Build history of the part. All positions in model axes, mm. Face numbers are marked on the shaded views. A direction names the side the tool comes from. Give positions to 0.01 mm unless a question says otherwise; leave off trailing zeros. Loops run counter-clockwise (first coordinate to the right, second up) from the corner with the lowest first, then second, coordinate; pieces in that order, holes last. Notation, with made-up numbers: (-34, 89) -> (-27, 89) arc R28 cw to (-27, 123) -> close; hole circle Ø8 at (-31, 84.25). An arc over 180 degrees is marked (long way). Answer as a JSON object with one key per item and string values. Group by question number.
Q1. Band-saw the part on B-B, the plane y = 9.75. Write the cut outline in (x, z), plus the area to 3 significant figures.
Q2. Band-saw the part on D-D, the plane x = 20. Write the cut outline in (y, z).
Q3. Band-saw the part on A-A, the plane x = 7. Write the cut outline in (y, z), plus the area to 3 significant figures.
Q4. Two-plate mould, pull along Y, no slides. Class the marked faces 4, 5 and 6: pulls with the +Y half, pulls with the -Y half, needs draft (parallel to the pull), parting line crosses it, or undercut.
Q5. Wall check: probe 1 along Y at (x, z) = (20, -4.85); probe 2 along X at (y, z) = (2.35, -5); probe 3 along X at (y, z) = (23, -8). Give the ranges that are in metal, low to high. Write a range as from..to.
Q6. Band-saw the part on C-C, the plane z = -6.25. Write the cut outline in (x, y), plus the area to 3 significant figures.
Q7. Drop flat-ended pins along their axis: pin 1 (2.5 mm diameter, centred on x = 20.5, z = -9, fed in from +Y); pin 2 (0.9 mm diameter, centred on y = 18, z = -8, fed in from +X); pin 3 (4.5 mm diameter, centred on x = 33, z = -5, fed in from +Y) (3 decimals); pin 4 (2.5 mm diameter, centred on y = 24, z = -8, fed in from -X). Give the stop position or say it passes through.
Q8. Tool access for the marked faces 1, 2 and 3: list every direction of +Z, -Z, +X, -X, +Y, -Y with a clear straight run to the whole face (end or side of a thin tool).
from build123d import *

# Parameters (mm, degrees)
SKETCH_1_W          = 40
SKETCH_1_H          = 10
EXTRUDE_1_DEPTH     = 3
SKETCH_2_W          = 13
SKETCH_2_H          = 3
EXTRUDE_2_DEPTH     = 43.75
EXTRUDE_3_DEPTH     = 3
RIB_1_REACH         = 62.314
SKETCH_5_WALL_W     = 166.48129864
SKETCH_5_WALL_H     = 2
RIB_START           = -2
RIB_2_DEPTH         = 2
SKETCH_8_R          = 1.6
CUT_EXTRUDE_1_DEPTH = 3
FILLET_1_R          = 2.5
SKETCH_9_R          = 2.45
SKETCH_9_R_2        = 2.5
CUT_EXTRUDE_5_DEPTH = 3
CHAMFER_2_SIZE      = 2


# Read off the part's stored shape, not the designer's step: the rib step
with BuildPart() as part:
    # Sketch 1 → Extrude 1 (new body)
    with BuildSketch(Plane(origin=(0, 0, 0), x_dir=(1, 0, 0), z_dir=(0, 1, 0))):
        with Locations((20, 5)):
            Rectangle(SKETCH_1_W, SKETCH_1_H)
    extrude(amount=EXTRUDE_1_DEPTH)

    # Sketch 2 → Extrude 2 (add)
    with BuildSketch(Plane(origin=(0, 3, 0), x_dir=(1, 0, 0), z_dir=(0, 1, 0))):
        with Locations((20, 5.5)):
            Rectangle(SKETCH_2_W, SKETCH_2_H)
    extrude(amount=EXTRUDE_2_DEPTH)

    # Sketch 4 → Extrude 3 (add)
    with BuildSketch(Plane.XY.offset(-4)):
        with BuildLine():
            Line((13.5, 46.75), (26.5, 46.75))
            ThreePointArc((26.5, 46.75), (20, 53.25), (13.5, 46.75))
        make_face()
    extrude(amount=-EXTRUDE_3_DEPTH)

    # Sketch 5 wall → Rib 1 (add, up to next)
    with BuildSketch(Plane(origin=(13.5, 24.875, -8.5), x_dir=(0, 0.997657238183, 0.068410782047), z_dir=(0, 0.068410782047, -0.997657238183)), mode=Mode.PRIVATE) as rib_1_sk1:
        with Locations((0, 1)):
            Rectangle(SKETCH_5_WALL_W, SKETCH_5_WALL_H)
    rib_1_tool1 = extrude(rib_1_sk1.sketch, amount=-RIB_1_REACH, mode=Mode.PRIVATE) - part.part
    add(rib_1_tool1.solids().sort_by_distance((13.5, 24.875, -8.5))[0])

    # Rib 2 outline → Rib 2 (add)
    with BuildSketch(Plane(origin=(26.5, 0, 0), x_dir=(0, 0, -1), z_dir=(1, 0, 0)).offset(RIB_START)):
        Polygon((10, 3), (7, 46.75), (7, 3), align=None)
    extrude(amount=RIB_2_DEPTH)

    # Sketch 8 → Cut-Extrude 1 (cut)
    with BuildSketch(Plane.XY.offset(-4)):
        with Locations((20, 9.75)):
            Circle(SKETCH_8_R)
        with Locations((20, 46.75)):
            Circle(SKETCH_8_R)
    extrude(amount=-CUT_EXTRUDE_1_DEPTH, mode=Mode.SUBTRACT)

    # Fillet 1
    fillet_1_edges = [part.edges().sort_by_distance(p)[0] for p in [
        (0, 1.5, -10),
        (40, 1.5, -10),
        (40, 1.5, 0),
        (0, 1.5, 0),
    ]]
    fillet(fillet_1_edges, radius=FILLET_1_R)

    # Sketch 9 → Cut-Extrude 5 (cut)
    with BuildSketch(Plane(origin=(0, 3, 0), x_dir=(1, 0, 0), z_dir=(0, 1, 0))):
        with Locations(Location((7, 5, 0), (0, 0, 270))):
            Circle(SKETCH_9_R)
        with Locations(Location((33, 5, 0), (0, 0, 270))):
            Circle(SKETCH_9_R_2)
    extrude(amount=-CUT_EXTRUDE_5_DEPTH, mode=Mode.SUBTRACT)

    # Chamfer 2
    chamfer_2_edges = [part.edges().sort_by_distance(p)[0] for p in [
        (13.5, 3, -7),
        (20, 3, -4),
        (26.5, 3, -7),
    ]]
    chamfer(chamfer_2_edges, length=CHAMFER_2_SIZE)


solid = part.part
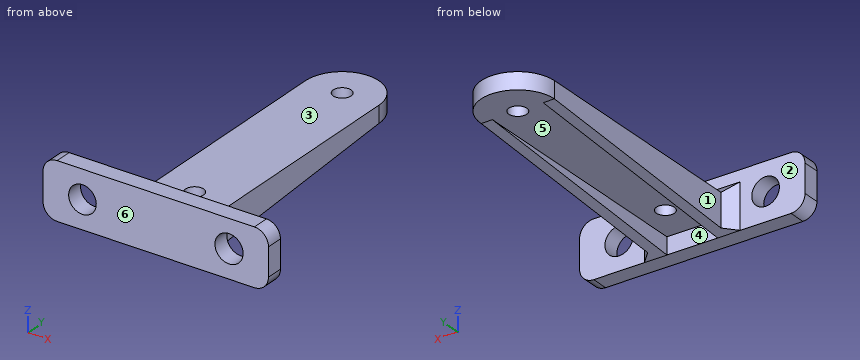
Worked answers:
{
 "1": {"outline": "(13.5, -9.54) -> (15.5, -9.54) -> (15.5, -7) -> (18.4, -7) -> (18.4, -4) -> (13.5, -4) -> close; (21.6, -7) -> (24.5, -7) -> (24.5, -9.54) -> (26.5, -9.54) -> (26.5, -4) -> (21.6, -4) -> close", "area": "39.5 mm2"},
 "2": {"outline": "(0, -10) -> (3, -10) -> (3, -7) -> (8.15, -7) -> (8.15, -4) -> (5, -4) -> (3, -2) -> (3, 0) -> (0, 0) -> close; (11.35, -7) -> (45.15, -7) -> (45.15, -4) -> (11.35, -4) -> close; (48.35, -7) -> (53.25, -7) -> (53.25, -4) -> (48.35, -4) -> close"},
 "3": {"outline": "(0, -10) -> (3, -10) -> (3, -7.45) -> (0, -7.45) -> close; (0, -2.55) -> (3, -2.55) -> (3, 0) -> (0, 0) -> close", "area": "15.3 mm2"},
 "4": {"face 4": "pulls with the +Y half", "face 5": "needs draft", "face 6": "pulls with the -Y half"},
 "5": {"probe 1": "0..8.15, 11.35..45.15, 48.35..53.25", "probe 2": "0..4.55, 9.45..30.5, 35.5..40", "probe 3": "13.5..15.5, 24.5..26.5"},
 "6": {"outline": "(0, 0) -> (4.89, 0) -> (4.89, 3) -> (0, 3) -> close; (9.11, 0) -> (30.83, 0) -> (30.83, 3) -> (28.5, 3) -> (26.5, 5) -> (26.5, 46.75) arc R6.5 ccw to (13.5, 46.75) -> (13.5, 5) -> (11.5, 3) -> (9.11, 3) -> close; (35.17, 0) -> (40, 0) -> (40, 3) -> (35.17, 3) -> close; hole circle Ø3.2 at (20, 9.75); hole circle Ø3.2 at (20, 46.75)", "area": "717 mm2"},
 "7": {"pin 1": "y = 3", "pin 2": "x = 26.5", "pin 3": "through", "pin 4": "x = 13.5"},
 "8": {"face 1": "+Z, -Z, -X, +Y", "face 2": "+Z, +Y", "face 3": "+Z, +X, -X, +Y"}
}
